Check sheet for the modelled part. Datum: model origin and axes. Units: mm. A direction names the side the tool comes from. Coordinates: 2 decimals unless noted, no trailing zeros. Loops run counter-clockwise (first coordinate to the right, second up) from the corner with the lowest first, then second, coordinate; pieces in that order, holes last. Notation, with made-up numbers: M -39.75,47.25 L 19.25,47.25 A26 cw 19.25,63.25 Z; hole C -0.75,67.5 d4. An arc over 180 degrees is marked long. Answer in a Markdown table with one row per item. Add a question column.
```python
from build123d import *

# Parameters (mm, degrees)
SKETCH_1_W          = 60
SKETCH_1_H          = 16
EXTRUDE_1_DEPTH     = 3
SKETCH_2_W          = 60
SKETCH_2_H          = 6
EXTRUDE_2_DEPTH     = 18
SKETCH_3_W          = 60
SKETCH_3_H          = 5
EXTRUDE_3_DEPTH     = 100
RIB_1_REACH         = 116.039
SKETCH_4_WALL_W     = 250.670193986
SKETCH_4_WALL_H     = 10
EXTRUDE_4_DEPTH     = 6
CUT_EXTRUDE_1_DEPTH = 115.039466852
SKETCH_8_3_R        = 15
CUT_EXTRUDE_2_DEPTH = 84.462566459


# Read off the part's stored shape, not the designer's step: 高级异型孔1
with BuildPart() as part:
    # 草图1 → 凸台-拉伸1 (new body)
    with BuildSketch(Plane(origin=(0, 0, 0), x_dir=(1, 0, 0), z_dir=(0, 1, 0))):
        Rectangle(SKETCH_1_W, SKETCH_1_H)
    extrude(amount=EXTRUDE_1_DEPTH)

    # 草图2 → 凸台-拉伸2 (add)
    with BuildSketch(Plane(origin=(0, 3, 0), x_dir=(1, 0, 0), z_dir=(0, 1, 0))):
        with Locations((0, -5)):
            Rectangle(SKETCH_2_W, SKETCH_2_H)
    extrude(amount=EXTRUDE_2_DEPTH)

    # 草图3 → 凸台-拉伸3 (add)
    with BuildSketch(Plane.XY.offset(8)):
        with Locations((0, 18.5)):
            Rectangle(SKETCH_3_W, SKETCH_3_H)
    extrude(amount=EXTRUDE_3_DEPTH)

    # 草图4 wall → 筋1 (add, up to next)
    with BuildSketch(Plane(origin=(0, 12, -3), x_dir=(0, -0.874157276122, -0.485642931179), z_dir=(0, 0.485642931179, -0.874157276122)), mode=Mode.PRIVATE) as rib_1_sk1:
        Rectangle(SKETCH_4_WALL_W, SKETCH_4_WALL_H)
    rib_1_tool1 = extrude(rib_1_sk1.sketch, amount=-RIB_1_REACH, mode=Mode.PRIVATE) - part.part
    add(rib_1_tool1.solids().sort_by_distance((0, 12, -3))[0])

    # 草图5 → 凸台-拉伸4 (add)
    with BuildSketch(Plane(origin=(30, 0, 0), x_dir=(0, 0, -1), z_dir=(1, 0, 0))):
        Polygon((-2, 21), (8, 3), (-2, 3), align=None)
    extrude_4 = extrude(amount=-EXTRUDE_4_DEPTH)

    # 镜向1: 凸台-拉伸4 across plane
    add(extrude_4.mirror(Plane(origin=(0, 0, 0), x_dir=(0, 0, 1), z_dir=(1, 0, 0))))

    # 高级异型孔1 outline → 高级异型孔1 (revolve, cut)
    with BuildSketch(Plane(origin=(-15, 0, -3), x_dir=(1, 0, 0), z_dir=(0, 0, 1))):
        Polygon((3.3, 3), (0, 3), (0, 0), (1.6, 0), (1.6, 1.3), align=None)
    other_1 = revolve(axis=Axis((-15, 0, -3), (0, 1, 0)), mode=Mode.SUBTRACT)

    # 镜向2: 高级异型孔1 across plane
    add(other_1.mirror(Plane(origin=(0, 0, 0), x_dir=(0, 0, 1), z_dir=(1, 0, 0))), mode=Mode.SUBTRACT)

    # 草图8 → 切除-拉伸1 (cut, through all)
    with BuildSketch(Plane(origin=(0, 21, 0), x_dir=(1, 0, 0), z_dir=(0, 1, 0))):
        with BuildLine():
            Line((-22.735407162, -55.478686702), (-30, -8))
            Line((-30, -8), (-30, -108))
            Line((-30, -108), (30, -108))
            Line((30, -108), (30, -8))
            Line((30, -8), (22.735407162, -55.478686702))
            ThreePointArc((22.735407162, -55.478686702), (0, -75), (-22.735407162, -55.478686702))
        make_face()
    extrude(amount=-CUT_EXTRUDE_1_DEPTH, mode=Mode.SUBTRACT)

    # 草图8<3> → 切除-拉伸2 (cut, through all)
    with BuildSketch(Plane(origin=(0, 21, 0), x_dir=(1, 0, 0), z_dir=(0, 1, 0))):
        with Locations(Location((0, -52, 0), (0, 0, 270))):
            Circle(SKETCH_8_3_R)
    extrude(amount=-CUT_EXTRUDE_2_DEPTH, mode=Mode.SUBTRACT)


solid = part.part
```
Q1. Mould release check, pull along X, two halves, no side actions. Record for faces 1 (the face through (24, 8, -1)), 2 (the face through (-30, 8, 2)), 3 (the face through (26.42, 18.54, 31.41)): released by +X, released by -X, zero draft, split by the parting line, or undercut.
Q2. Cross-section at D-D (z = 52). Record the cut outline in (x, y).
Q3. Access from +Z, -Z, +X, -X, +Y, -Y to the whole of each face (thin tool, end or side, straight path). Record for faces 4 (the face through (-24, 8, -1)), 5 (the face through (-16.705, 1.406, -3.075)), 6 (the face through (0, 8, 8)).
Q4. Cross-section at A-A (x = 0). Record the cut outline in (y, z), plus the area to 3 significant figures.
Q5. Thickness scan on L1, parallel to X at y = 0.55, z = -3; L2, parallel to Z at x = 15, y = 0.9; L3, parallel to Y at x = 10.5, z = 63. Record the ranges inside material, lowest first.
Q6. Go/stop test with flat-tipped pins: pin 1 (8 mm diameter, centred on y = 17, z = 30.5, fed in from -X); pin 2 (5 mm diameter, centred on x = -9, y = 10, fed in from +Z); pin 3 (18 mm diameter, centred on x = 0, z = 52, fed in from -Y); pin 4 (6 mm diameter, centred on x = -4.5, y = 14, fed in from +Z). Record where each tip stops, or that it passes through.
Q7. Cross-section at C-C (y = 7.5). Record the cut outline in (x, z).
Q8. Cross-section at B-B (z = -3). Record the cut outline in (x, y).
Answer key:
| question | item | result |
|---|---|---|
| 1 | face 1 | undercut |
| 1 | face 2 | released by -X |
| 1 | face 3 | released by +X |
| 2 | outline | M -23.27,16 L -15,16 L -15,21 L -23.27,21 Z; M 15,16 L 23.27,16 L 23.27,21 L 15,21 Z |
| 3 | face 4 | -Z, +Y |
| 3 | face 5 | +Y |
| 3 | face 6 | +Z, +X, -X, -Y |
| 4 | outline | M 0,-8 L 3,-8 L 21,2 L 21,37 L 16,37 L 16,8 L 0,8 Z; M 16,67 L 21,67 L 21,75 L 16,75 Z |
| 4 | area | 431 mm^2 |
| 5 | L1 | -30 to -16.6, -13.4 to 13.4, 16.6 to 30 |
| 5 | L2 | -8 to -4.6, -1.4 to 8 |
| 5 | L3 | 16 to 21 |
| 6 | pin 1 | x = -27.17 |
| 6 | pin 2 | z = 8 |
| 6 | pin 3 | through |
| 6 | pin 4 | z = 74.89 |
| 7 | outline | M -30,-5.5 L -24,-5.5 L -24,2 L -5,2 L -5,-5.5 L 5,-5.5 L 5,2 L 24,2 L 24,-5.5 L 30,-5.5 L 30,8 L -30,8 Z |
| 8 | outline | M -30,0 L -16.6,0 L -16.6,1.3 L -18.3,3 L -24,3 L -24,12 L -30,12 Z; M -13.4,0 L 13.4,0 L 13.4,1.3 L 11.7,3 L 5,3 L 5,12 L -5,12 L -5,3 L -11.7,3 L -13.4,1.3 Z; M 16.6,0 L 30,0 L 30,12 L 24,12 L 24,3 L 18.3,3 L 16.6,1.3 Z |
